For this review, take the finished solid that the model builds, in its own axes (mm). Coordinates: 2 decimals unless noted, no trailing zeros. Loops run counter-clockwise (first coordinate to the right, second up) from the corner with the lowest first, then second, coordinate; pieces in that order, holes last. Notation, with made-up numbers: (23, 34.25) -> (73, 34.25) arc R22 ccw to (73, 59.25) -> close; hole circle Ø7 at (-10, 89.5). An arc over 180 degrees is marked (long way). Use a Markdown table: item, result.
Autodesk Inventor part; units mm, degrees
ref_plane "YZ Plane" through (0, 0, 0) normal (1, 0, 0) x (0, 1, 0)
ref_plane "XZ Plane" through (0, 0, 0) normal (0, 1, 0) x (-1, 0, 0)
ref_plane "XY Plane" through (0, 0, 0) normal (0, 0, 1) x (1, 0, 0)
sketch "Sketch1" plane through (0, 0, 0) normal (0, 1, 0) x (-1, 0, 0)
  line L0 (0, 0) -> (200, 0)
  line L1 (200, 0) -> (200, -7.5533)
  line L2 (180, -20) -> (0, -20)
  line L3 (0, -20) -> (0, 0)
  line L4 (200, 0) -> (180, -20)
  line L5 (182.0213, -10) -> (194.6749, -10)
  line L6 (182.4568, -14.0077) -> (191.5424, -4.9221)
  line L7 (182.4568, -14.0077) -> (184.7026, -15.2974)
  line L8 (191.5424, -4.9221) -> (193.7882, -6.2118)
  point P0 (200, -10)
  dimension "d0" = 20
  dimension "d1" = 200
  dimension "d7" = 10
  dimension "d8" = 2.5
  dimension "d9" = 12.849
extrude "Extrusion1" add sketch "Sketch1" along normal blind 5 contours L0 L4 L8 L6 L7 L2 L3
properties part number "Yaxix" material "Wood (Birch)"
(1) Take a section at A-A on y = 3.25. Write out the cut boundary in (x, z).
Found:
| item | result |
|---|---|
| outline | (-200, 0) -> (-193.79, -6.21) -> (-191.54, -4.92) -> (-182.46, -14.01) -> (-184.7, -15.3) -> (-180, -20) -> (0, -20) -> (0, 0) -> close |
(2) Take a section at B-B on z = -17.25. Write out the cut boundary in (x, y).
Found:
| item | result |
|---|---|
| outline | (-182.75, 0) -> (0, 0) -> (0, 5) -> (-182.75, 5) -> close |
(3) Mouldability with a two-part tool opening along Z and no side actions: class faces 1 (the face through (-99, 5, -10)), 2 (the face through (-99, 2, 0)), 3 (the face through (-186.936, 2.465, -9.528)) as pulls with the +Z half, pulls with the -Z half, needs draft (parallel to the pull), parting line crosses it, or undercut.
Found:
| item | result |
|---|---|
| face 1 | needs draft |
| face 2 | pulls with the +Z half |
| face 3 | undercut |
(4) For line 1 along X through (y, z) = (1.3, -11.75); line 2 along X through (y, z) = (4.85, -5.25); line 3 along X through (y, z) = (2.3, -14), list the stretches that pass through material, from the lowest coordinate up.
Found:
| item | result |
|---|---|
| line 1 | x = -184.71 to 0 |
| line 2 | x = -194.75 to -192.11, -191.21 to 0 |
| line 3 | x = -182.46 to 0 |
